Print and shaded views of the part. All mm, measured from the part's lowest x, y and z. A direction names the side the tool comes from. Coordinates: 2 decimals unless noted, no trailing zeros. Order: outer loops, then holes, each group sorted by start corner. A loop starts at its lowest first (then second) coordinate and runs counter-clockwise, first axis right, second up. Notation, with made-up numbers: (37, 8) -> (76, 8) arc R25 cw to (76, 25) -> close; hole circle Ø5 at (73, 44). An arc over 180 degrees is marked (long way). Write item = value, one per line. Start each with the question number.
Q1. Cut at C-C, the plane y = 7.5. List the corners of the cut face in (x, z), plus the area to 3 significant figures.
Q2. Cut at D-D, the plane x = 26. List the corners of the cut face in (y, z).
Q3. 3-axis set-ups, long thin cutter, end or side, ignore diameter. For the marked faces 1 and 2: which of +Z, -Z, +X, -X, +Y, -Y reach the whole face in a straight line?
Q4. Mould opens along X. For the marked faces 3, 4 and 5 say: +X half, -X half, draft (parallel to the pull), parting line (faces both ways), or undercut.
Q5. Cut at B-B, the plane x = 16.85. List the corners of the cut face in (y, z), plus the area to 3 significant figures.
Q6. Flat gauge pins, fed straight in: pin 1 (3 mm diameter, centred on x = 14, y = 3.5, fed in from -Z); pin 2 (5 mm diameter, centred on y = 9, z = 9.5, fed in from +X). Where does each tip first touch, or does it go through?
Q7. Wall check: line 1 (X direction, y = 10.9, z = 16.85); line 2 (X direction, y = 6.75, z = 77.81); line 3 (X direction, y = 8.25, z = 16.85). Give the ranges that are in metal, low to high. Write a range as from..to.
Q8. Cut at A-A, the plane y = 1. List the corners of the cut face in (x, z).
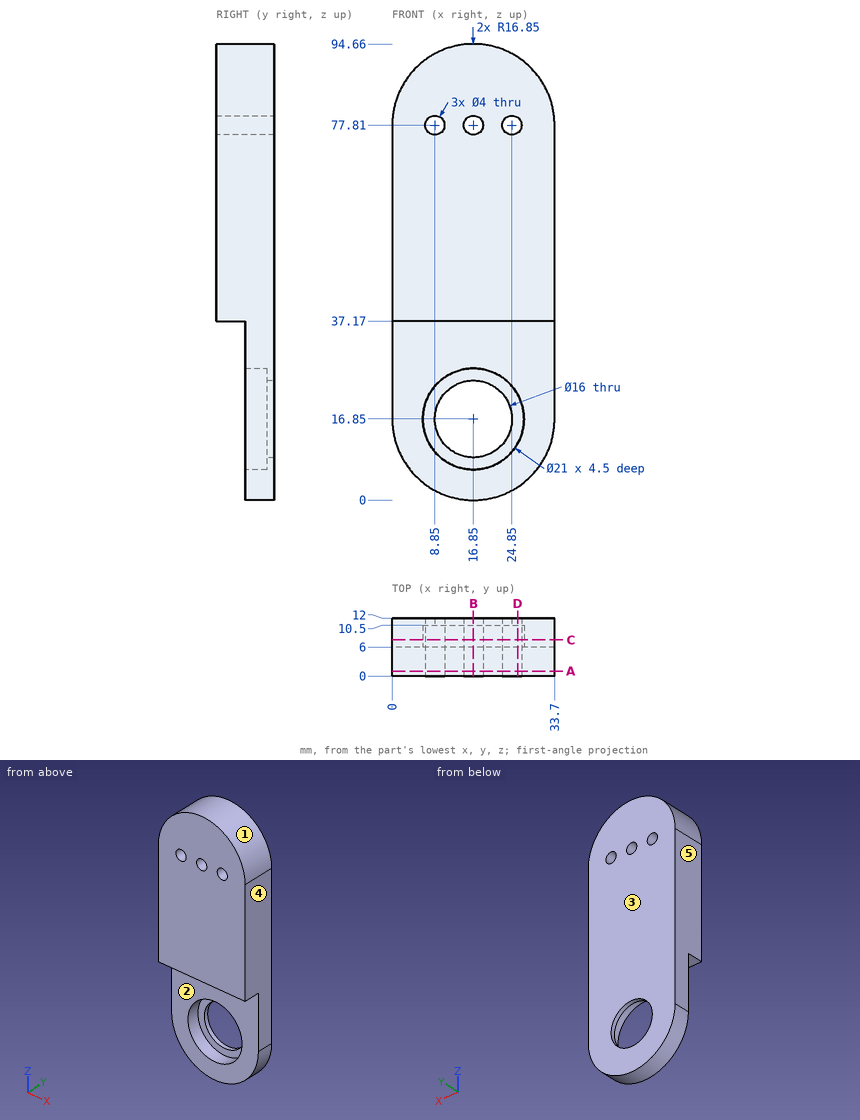
Here are the results:
q1.outline = (0, 16.85) arc R16.85 ccw to (33.7, 16.85) -> (33.7, 77.81) arc R16.85 ccw to (0, 77.81) -> close; hole circle Ø21 at (16.85, 16.85); hole circle Ø4 at (8.85, 77.81); hole circle Ø4 at (16.85, 77.81); hole circle Ø4 at (24.85, 77.81)
q1.area = 2,560 mm²
q2.outline = (0, 37.17) -> (6, 37.17) -> (6, 22) -> (10.5, 22) -> (10.5, 11.7) -> (6, 11.7) -> (6, 2.7) -> (12, 2.7) -> (12, 76.17) -> (0, 76.17) -> close; (0, 79.45) -> (12, 79.45) -> (12, 91.96) -> (0, 91.96) -> close
q3.face_1 = +Z, +Y, -Y
q3.face_2 = -Z, +X, -X, -Y
q4.face_3 = draft
q4.face_4 = +X half
q4.face_5 = -X half
q5.outline = (0, 37.17) -> (6, 37.17) -> (6, 27.35) -> (10.5, 27.35) -> (10.5, 24.85) -> (12, 24.85) -> (12, 75.81) -> (0, 75.81) -> close; (0, 79.81) -> (12, 79.81) -> (12, 94.66) -> (0, 94.66) -> close; (6, 0) -> (12, 0) -> (12, 8.85) -> (10.5, 8.85) -> (10.5, 6.35) -> (6, 6.35) -> close
q5.area = 746 mm²
q6.pin_1 = 37.17
q6.pin_2 = 32.99
q7.line_1 = 0..8.85, 24.85..33.7
q7.line_2 = 0..6.85, 10.85..14.85, 18.85..22.85, 26.85..33.7
q7.line_3 = 0..6.35, 27.35..33.7
q8.outline = (0, 37.17) -> (33.7, 37.17) -> (33.7, 77.81) arc R16.85 ccw to (0, 77.81) -> close; hole circle Ø4 at (8.85, 77.81); hole circle Ø4 at (16.85, 77.81); hole circle Ø4 at (24.85, 77.81)
